The listing builds one solid part. Answer for the finished solid, in the listing's coordinates (mm). Give positions to 0.01 mm unless a question says otherwise; leave off trailing zeros. Write each loop counter-clockwise with the first axis right and the second up, starting at its lowest first coordinate (ties: lowest second). Pieces come first, ordered by that corner, then holes. Notation, with made-up numbers: M 84.5,58.25 L 108.5,58.25 A25 ccw 108.5,84.25 Z; hole C 63,-27.75 d7. An arc over 180 degrees is marked long. Answer as a JSON object with one key per item and string values.
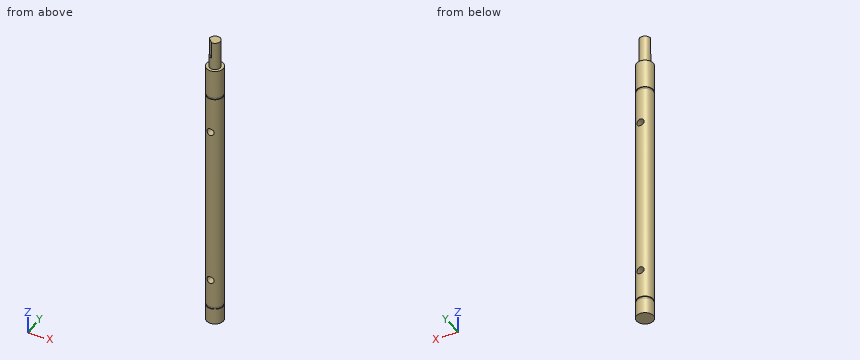
```python
from build123d import *

# Parameters (mm, degrees)
SKETCH1_W                 = 3.175
SKETCH1_H                 = 9.525
SKETCH1_H_2               = 50.8
F_6_32_TAPPED_HOLE1_D     = 2.7051
F_6_32_TAPPED_HOLE1_DEPTH = 9.398
F_6_32_TAPPED_HOLE1_TIP   = 0.81269403
CUT_EXTRUDE1_DEPTH        = 6.35


with BuildPart() as part:
    # Sketch1 → Revolve1 (revolve)
    with BuildSketch(Plane(origin=(0, 0, 0), x_dir=(1, 0, 0), z_dir=(0, 1, 0)), mode=Mode.PRIVATE) as revolve1_sk:
        Polygon((-38.708137827, 86.94610411), (-35.533137827, 86.94610411), (-35.533137827, 99.795553682), (-38.708137827, 99.795553682), (-38.708137827, 93.769403682), (-38.454137827, 93.769403682), (-38.454137827, 93.032803682), (-38.708137827, 93.032803682), align=None)
        with Locations((-37.120637827, 82.18360411)):
            Rectangle(SKETCH1_W, SKETCH1_H)
        with Locations((-37.120637827, 52.02110411)):
            Rectangle(SKETCH1_W, SKETCH1_H_2)
        with Locations((-37.120637827, 21.85860411)):
            Rectangle(SKETCH1_W, SKETCH1_H)
        Polygon((-38.708137827, -3.175), (-37.583137827, -3.175), (-37.583137827, -13.843), (-35.533137827, -13.843), (-35.533137827, 17.09610411), (-38.708137827, 17.09610411), (-38.708137827, 8.3566), (-38.454137827, 8.3566), (-38.454137827, 7.62), (-38.708137827, 7.62), align=None)
    revolve(revolve1_sk.sketch.rotate(Axis((-35.533137827, 0, 13.843), (0, 0, -1)), 180), axis=Axis((-35.533137827, 0, 13.843), (0, 0, -1)))

    # #6-32 Tapped Hole1
    with Locations(Plane(origin=(0, -3.175, 0), x_dir=(-1, 0, 0), z_dir=(0, -1, 0))):
        with Locations((35.533137827, 82.18360411), (35.533137827, 21.85860411)):
            Hole(F_6_32_TAPPED_HOLE1_D / 2, depth=F_6_32_TAPPED_HOLE1_DEPTH)
            with Locations((0, 0, -(F_6_32_TAPPED_HOLE1_DEPTH + F_6_32_TAPPED_HOLE1_TIP / 2))):  # 118° drill point
                Cone(0, F_6_32_TAPPED_HOLE1_D / 2, F_6_32_TAPPED_HOLE1_TIP, mode=Mode.SUBTRACT)

    # Sketch4 → Cut-Extrude1 (cut)
    with BuildSketch(Plane.XY.offset(13.843)):
        Polygon((-19.85306803, -17.854423149), (-35.661514798, -2.045976381), (-37.579114208, -0.128376971), (-53.387560976, 15.680069797), (-85.00445451, -15.936823738), (-51.469961565, -49.471316683), align=None)
    extrude(amount=-CUT_EXTRUDE1_DEPTH, mode=Mode.SUBTRACT)


solid = part.part
```
1. A cutting plane is placed at A-A, the plane z = -56. Give the vertices of the cut face in (x, y) (3 decimals), plus the area to 3 significant figures.
Verdict:
{"outline": "C -35.533,0 d6.35", "area": "31.7 mm2"}
2. Consider line 1 along Z through (x, y) = (-36.75, -1); line 2 along Z through (x, y) = (-37, 2.25) (3 decimals); line 3 along Z through (x, y) = (-34.75, 0). Determine where each line is inside the solid, lowest interval first.
Verdict:
{"line 1": "z = -99.8 to -82.77, -81.59 to -22.45, -21.27 to 7.49", "line 2": "z = -99.796 to 3.175", "line 3": "z = -99.8 to -83.29, -81.08 to -22.96, -20.76 to 13.84"}
3. Flat-ended cylindrical pins translate along their axes: pin 1 (3 mm diameter, centred on x = -34.5, z = -21, fed in from +Y) (3 decimals); pin 2 (2.5 mm diameter, centred on x = -35.53, z = -82.18, fed in from -Y); pin 3 (1.5 mm diameter, centred on x = -37.5, z = -66.5, fed in from +Y). Find the tip coordinate at first contact, or state that the pin passes through.
Verdict:
{"pin 1": "stops at y = 3.175", "pin 2": "passes through", "pin 3": "stops at y = 2.93"}
